Check sheet for the drawn part. Datum: minimum x, y, z corner. Units: mm. A direction names the side the tool comes from. Coordinates: 2 decimals unless noted, no trailing zeros. Loops run counter-clockwise (first coordinate to the right, second up) from the corner with the lowest first, then second, coordinate; pieces in that order, holes last. Notation, with made-up numbers: (-17.5, 19.25) - (1.5, 19.25) arc R12 ccw to (1.5, 37.25) - close; hole circle Ø10 at (14, 23). An arc over 180 degrees is marked (long way). Answer as CSV lines item,"result". Start each with the question number.
1. Material ranges on line 1 (Y direction, x = 73.5, z = 33); line 2 (X direction, y = 35, z = 22.5); line 3 (X direction, y = 37, z = 6), recorded low to high. Write a range as [from, to].
2. Set-up check for the marked faces 1, 2 and 3: record each of +Z, -Z, +X, -X, +Y, -Y from which the full face is reachable in a straight line by a thin tool's end or side.
3. Release check for a two-part mould opening along Y. For the marked faces 4, 5, 6 and 7 record: pulls with the +Y half, pulls with the -Y half, needs draft (parallel to the pull), parting line crosses it, or undercut.
4. Gauge pin test, flat ends, axial feed: P1, Ø1, axis at y = 44.5, z = 44.5, coming from the -X side; P2, Ø24, axis at y = 22.5, z = 25, coming from the +X side. Record the tip position at first contact, or that the pin passes through.
5. Cross-section at D-D (z = 15). Enter the section's corners in (x, y).
6. Cross-section at B-B (y = 45.5). Enter the section's corners in (x, z).
7. Cross-section at C-C (x = 43). Enter the section's corners in (y, z), plus the area to 3 significant figures.
8. Cross-section at A-A (z = 43). Enter the section's corners in (x, y), plus the area to 3 significant figures.
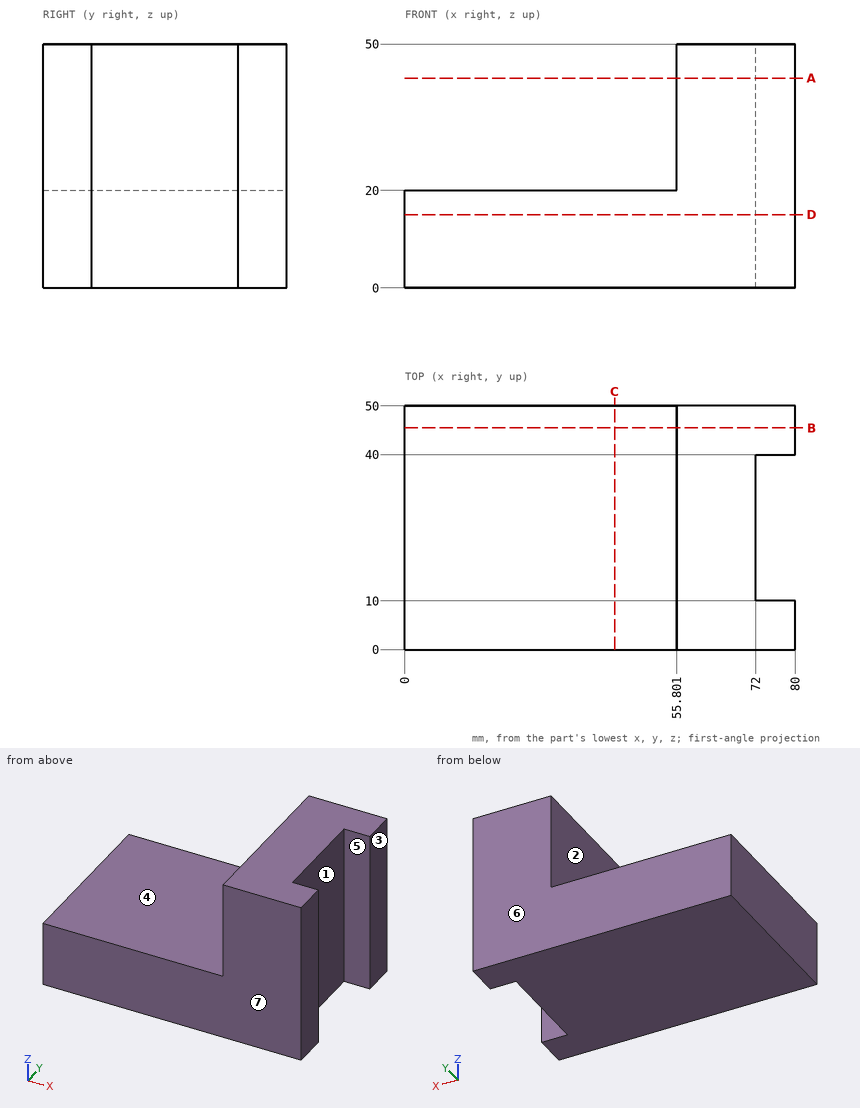
Values follow:
1,line 1,"y = [0, 10], [40, 50]"
1,line 2,"x = [55.8, 72]"
1,line 3,"x = [0, 72]"
2,face 1,"+Z, -Z, +X"
2,face 2,"+Z, -X, +Y, -Y"
2,face 3,"+Z, -Z, +X, +Y, -Y"
3,face 4,"needs draft"
3,face 5,"undercut"
3,face 6,"pulls with the +Y half"
3,face 7,"pulls with the -Y half"
4,P1,"stops at x = 55.8"
4,P2,"stops at x = 72"
5,outline,"(0, 0) - (80, 0) - (80, 10) - (72, 10) - (72, 40) - (80, 40) - (80, 50) - (0, 50) - close"
6,outline,"(0, 0) - (80, 0) - (80, 50) - (55.8, 50) - (55.8, 20) - (0, 20) - close"
7,outline,"(0, 0) - (50, 0) - (50, 20) - (0, 20) - close"
7,area,"1,000 mm²"
8,outline,"(55.8, 0) - (80, 0) - (80, 10) - (72, 10) - (72, 40) - (80, 40) - (80, 50) - (55.8, 50) - close"
8,area,"970 mm²"
